Autodesk Inventor part; units mm, degrees
ref_plane "YZ Plane" through (0, 0, 0) normal (1, 0, 0) x (0, 1, 0)
ref_plane "XZ Plane" through (0, 0, 0) normal (0, 1, 0) x (-1, 0, 0)
ref_plane "XY Plane" through (0, 0, 0) normal (0, 0, 1) x (1, 0, 0)
sketch "Эскиз1" plane through (0, 0, 0) normal (0, 0, 1) x (1, 0, 0)
  circle A0 centre (0, 0) radius 3.5
  dimension "d0" = 7
extrude "Выдавливание1" add sketch "Эскиз1" along normal blind 7
fillet "Сопряжение1" radius 2 1 edges at (-3.5, 0, 7)
sketch "Эскиз2" plane through (0, 0, 0) normal (0, 0, -1) x (-1, 0, 0)
  circle A0 centre (0, 0) radius 1.5
  circle A1 centre (0, 0) radius 1.5
  dimension "d4" = 3
extrude "Выдавливание2" cut sketch "Эскиз2" against normal blind 5.8
properties part number "back_pimp"
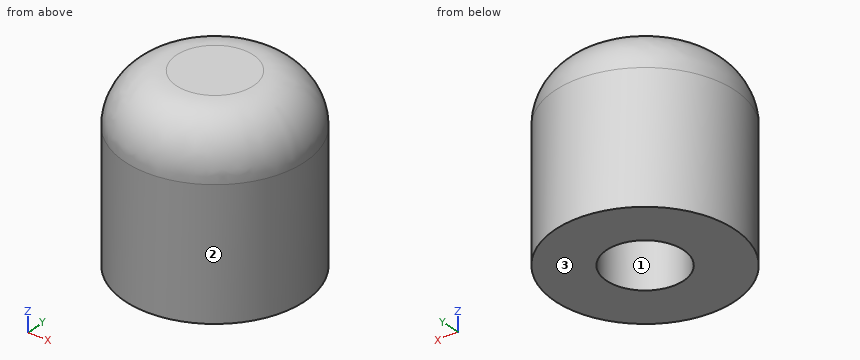
The model under review builds one solid part; all positions refer to its coordinate system, in mm. Face numbers are marked on the shaded views. Round coordinates to 2 decimals unless told otherwise and drop trailing zeros. Order: outer loops, then holes, each group sorted by start corner. A loop starts at its lowest first (then second) coordinate and runs counter-clockwise, first axis right, second up. Notation, with made-up numbers: (-29.5, -23) -> (-18.5, -23) arc R23 ccw to (-18.5, 5) -> close; hole circle Ø2 at (50.5, 59). An arc over 180 degrees is marked (long way). One line per item, written item: value. Start each with the question number.
Q1. Take a section at A-A (z = 1.25). Write out the cut boundary in (x, y), and give its area (3 significant figures).
Q2. Wall thickness on line 1 (Y direction, x = 0, z = 1.45); line 2 (X direction, y = 0.75, z = 4.25); line 3 (Z direction, x = 0.25, y = 1): over which ranges is each line inside the solid? List them lowest first.
Q3. Mouldability with a two-part tool opening along Y and no side actions: class the marked faces 1, 2 and 3 as released by +Y, released by -Y, zero draft, split by the parting line, or undercut.
Reported:
1. outline: circle Ø7 at (0, 0); hole circle Ø3 at (0, 0)
1. area: 31.4 mm2
2. line 1: y = -3.5 to -1.5, 1.5 to 3.5
2. line 2: x = -3.42 to -1.3, 1.3 to 3.42
2. line 3: z = 5.8 to 7
3. face 1: undercut
3. face 2: split by the parting line
3. face 3: zero draft
